Autodesk Inventor part; units mm, degrees
ref_plane "YZ Plane" through (0, 0, 0) normal (1, 0, 0) x (0, 1, 0)
ref_plane "XZ Plane" through (0, 0, 0) normal (0, 1, 0) x (-1, 0, 0)
ref_plane "XY Plane" through (0, 0, 0) normal (0, 0, 1) x (1, 0, 0)
sketch "Skizze1" plane through (0, 0, 0) normal (0, 0, 1) x (1, 0, 0)
  line L0 (-220, -220) -> (220, -220)
  line L1 (220, 220) -> (220, -220)
  line L2 (-220, 220) -> (-220, -220)
  line L3 (-220, 220) -> (220, 220)
  line L4 (200, 200) -> (-200, 200)
  line L5 (-200, 200) -> (-200, -200)
  line L6 (-200, -200) -> (200, -200)
  line L7 (200, -200) -> (200, 200)
  line L8 (220, -220) -> (-220, -220)
  line L9 (-220, -220) -> (-220, 220)
  line L10 (-220, 220) -> (220, 220)
  line L11 (220, 220) -> (220, -220)
  line L12 (200, -200) -> (-200, -200)
  line L13 (-200, -200) -> (-200, 200)
  line L14 (-200, 200) -> (200, 200)
  line L15 (200, 200) -> (200, -200)
  point P0 (0, 0)
extrude "Extrusion1" add sketch "Skizze1" against normal blind 20
chamfer "Fase1" distance 20 angle 45 4 edges at (220, 0, -20) (0, 220, -20) (0, -220, -20) (-220, 0, -20)
ref_plane "Arbeitsebene1" through (0, 0, -20) normal (0, 0, 1) x (1, 0, 0)
sketch "Skizze3" plane through (0, 0, -20) normal (0, 0, 1) x (1, 0, 0)
  arc A0 (-205, 25.5) -> (-205, 4.5) centre (-205, 15) ccw
  arc A1 (-205, 25.5) -> (-205, 4.5) centre (-205, 15) ccw
  arc A2 (-205, -5.9522) -> (-205, -26.9522) centre (-205, -16.4522) ccw
  arc A3 (-205, -5.9522) -> (-205, -26.9522) centre (-205, -16.4522) ccw
  arc A4 (-205, -5.9522) -> (-205, -26.9522) centre (-205, -16.4522) ccw
  arc A5 (-205, -5.9522) -> (-205, -26.9522) centre (-205, -16.4522) ccw
  line L0 (-200, -26.9522) -> (-205, -26.9522)
  line L1 (-205, -5.9522) -> (-200, -5.9522)
  line L2 (-205, 4.5) -> (-200, 4.5)
  line L3 (-200, -200) -> (-200, 200)
  line L4 (-205, 25.5) -> (-200, 25.5)
  line L5 (-205, -5.9522) -> (-200, -5.9522)
  line L6 (-205, -26.9522) -> (-200, -26.9522)
  arc A6 (-205, 25.5) -> (-205, 4.5) centre (-205, 15) ccw
  arc A7 (-205, -5.9522) -> (-205, -26.9522) centre (-205, -16.4522) ccw
  point P0 (0, 0)
extrude "Extrusion2" cut sketch "Skizze3" along normal blind 17
sketch "Skizze5" plane through (0, 0, -20) normal (0, 0, 1) x (1, 0, 0)
  line L0 (-200, -26.9522) -> (-200, -200)
  line L1 (-200, -200) -> (200, -200)
  line L2 (200, -200) -> (200, 200)
  line L3 (-200, 200) -> (200, 200)
  line L4 (-200, -200) -> (200, -200)
  line L5 (200, -200) -> (200, 200)
  line L6 (200, 200) -> (-200, 200)
  line L7 (-200, 200) -> (-200, -200)
  line L8 (-190, -190) -> (190, -190)
  line L9 (190, -190) -> (190, 190)
  line L10 (190, 190) -> (-190, 190)
  line L11 (-190, 190) -> (-190, -190)
  point P0 (0, 0)
  dimension "d8" = 10
  dimension "d9" = 10
  dimension "d10" = 10
  dimension "d11" = 10
extrude "Extrusion3" add sketch "Skizze5" along normal blind 10
properties part number "PV_Ramen_CPY_3_2"
Build history of the part. All positions in model axes, mm. A direction names the side the tool comes from. Round coordinates to 2 decimals unless told otherwise and drop trailing zeros. One line per item, written item: value. Start each with the question number.
Q1. Cut at C-C on y = 15. Count the separate pieces of the cut face and the enclosed holes in it, plus the area to 3 significant figures.
Q2. Two-plate mould, pull along Y, no slides. Class faces 4 (the face through (-3, -210, -10)), 5 (the face through (-3, -200, -5)), 6 (the face through (-16, -192, -20)): released by +Y, released by -Y, zero draft, split by the parting line, or undercut.
Q3. 3-axis set-ups, long thin cutter, end or side, ignore diameter. For faces 1 (the face through (-16, -192, -10)), 2 (the face through (-215.497, -16.683, -3.751)), 3 (the face through (-190, 3, -15)): which of +Z, -Z, +X, -X, +Y, -Y reach the whole face in a straight line?
Q4. Drop flat-ended pins along their axis: pin 1 Ø12 at (y, z) = (-55.5, -9) entering from -X; pin 2 Ø8 at (y, z) = (4.5, -4.5) entering from +X; pin 3 Ø2 at (y, z) = (-9.5, -14.5) entering from +X. Give the stop position or say it passes through.
Q5. Probe line 1 along Y through (x, z) = (136.5, -14); line 2 along X through (y, z) = (-174.5, -17); line 3 along Y through (x, z) = (-158.5, -18). List the from-to ranges inside material, lowest first.
Computed:
1. separate pieces: 3
1. enclosed holes: 0
1. area: 457 mm²
2. face 4: released by -Y
2. face 5: undercut
2. face 6: zero draft
3. face 1: +Z
3. face 2: -Z
3. face 3: +Z, -Z
4. pin 1: x = -217
4. pin 2: x = 219.5
4. pin 3: x = 206.5
5. line 1: -206 to -190, 190 to 206
5. line 2: -203 to -190, 190 to 203
5. line 3: -202 to -190, 190 to 202
